Here's how the part is built. I have some questions about the finished solid (model axes, mm). Face numbers are marked on the shaded views. A direction names the side the tool comes from. Give positions to 0.01 mm unless a question says otherwise; leave off trailing zeros. Loops run counter-clockwise (first coordinate to the right, second up) from the corner with the lowest first, then second, coordinate; pieces in that order, holes last.
Q1. For the marked faces 1 and 2, which set-ups out of +Z, -Z, +X, -X, +Y, -Y let a thin tool reach every point of the face, with its end or its side?
Q2. Suppose I cut it at A-A (x = -25). List the corners of the cut face in (y, z) for me.
Q3. Suppose I cut it at D-D (y = -60.5). List the corners of the cut face in (x, z) for me, and give its area (3 significant figures).
Q4. Thinking about a two-plate mould opening in Z: for the marked faces 3, 4 and 5, which applies, pulls with the +Z half, pulls with the -Z half, needs draft (parallel to the pull), parting line crosses it, or undercut?
Q5. Suppose I cut it at C-C (z = -34). List the corners of the cut face in (x, y) for me, and give its area (3 significant figures).
Q6. I'm going to push flat-ended pins straight in: P1, Ø9, axis at x = -25, z = 0, coming from the +Y side; P2, Ø11, axis at x = 44.5, z = -45.5, coming from the +Y side; P3, Ø8, axis at x = 68.5, z = -7, coming from the -Y side; P4, Ø9, axis at x = 0, y = 0, coming from the -Z side. Where does each tip first touch, or does it pass through?
Q7. I need wall thicknesses on probe 1 along Y at (x, z) = (0, -49); probe 2 along Z at (x, y) = (-17, -44); probe 3 along X at (y, z) = (19.5, -35). Which ranges of each line are inside material? Lowest first, please.
Q8. Suppose I cut it at B-B (y = 35.5). List the corners of the cut face in (x, z) for me.
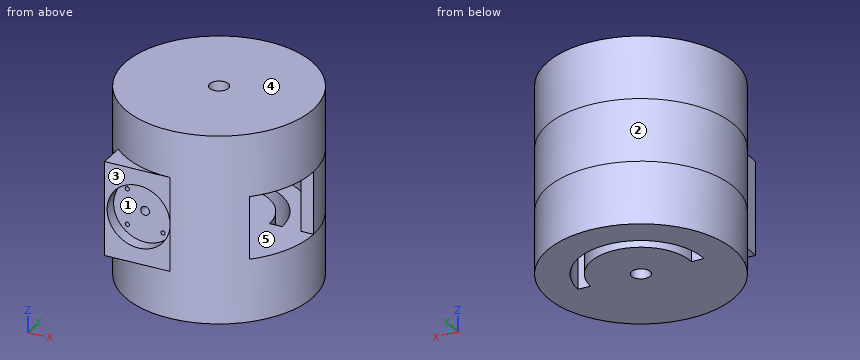
Autodesk Inventor part; units mm, degrees
ref_plane "Work Plane4" through (0, 0, 0) normal (0, 0, -1) x (-1, 0, 0)
ref_plane "YZ Plane" through (0, 0, 0) normal (1, 0, 0) x (0, 1, 0)
ref_plane "XZ Plane" through (0, 0, 0) normal (0, 1, 0) x (-1, 0, 0)
sketch "Sketch1" plane through (0, 0, 0) normal (0, 0, 1) x (1, 0, 0)
  circle A0 centre (0, 0) radius 75
  dimension "d0" = 150
extrude "Extrusion1" add sketch "Sketch1" along normal mid plane 150
sketch "Sketch32" plane through (0, 0, 0) normal (0, 0, 1) x (1, 0, 0)
  line L0 (0, 0) -> (-52, 0)
  line L1 (-52, 0) -> (-52, -75)
  line L2 (-52, -75) -> (0, -75)
  line L3 (0, -75) -> (0, 0)
  dimension "d94" = 52
  dimension "d95" = 75
extrude "Extrusion23" add sketch "Sketch32" along normal mid plane 75
sketch "Sketch39" plane through (0, 0, -75) normal (0, 0, -1) x (-1, 0, 0)
  circle A0 centre (0, 0) radius 7.5
  dimension "d141" = 15
extrude "Extrusion30" cut sketch "Sketch39" against normal through all
ref_plane "Work Plane4" through (0, 0, 0) normal (0, 0, -1) x (-1, 0, 0)
sketch "Sketch40" plane through (0, 0, 0) normal (0, 0, -1) x (-1, 0, 0)
  circle A0 centre (0, 0) radius 75
  dimension "d144" = 150
extrude "Extrusion31" cut sketch "Sketch40" along normal mid plane 50
sketch "Sketch41" plane through (0, 0, 0) normal (0, 0, -1) x (-1, 0, 0)
  line L0 (52, -75) -> (52, -54.0463)
  line L1 (52, -54.0463) -> (-52, -54.0463)
  circle A0 centre (0, 0) radius 75
  arc A1 (-52, -54.0463) -> (0, -75) centre (0, 0) ccw
extrude "Extrusion32" add sketch "Sketch41" along normal mid plane 50 contours A0 L1 picked at (-14.3807, -56.4807)
sketch "Sketch34" plane through (-52, -75, 37.5) normal (0, -1, 0) x (1, 0, 0)
  circle A0 centre (27, -37.5) radius 25
  line L0 (52, -75) -> (0, -75)
  line L1 (-23, -112.5) -> (127, -112.5)
  point P0 (52, -37.5)
  dimension "d104" = 50
  dimension "d105" = 25
  dimension "d106" = 37.5
extrude "Extrusion25" cut sketch "Sketch34" against normal blind 10
sketch "Sketch42" plane through (0, 0, 0) normal (0, 0, -1) x (-1, 0, 0)
  arc A0 (47, -44.8999) -> (1.9436, 64.9709) centre (0, 0) ccw
  line L0 (47, -44.8999) -> (47, -54.0463)
  line L1 (47, -54.0463) -> (52, -54.0463)
  arc A1 (52, -54.0463) -> (-75, 0) centre (0, 0) ccw
  arc A2 (47, -44.8999) -> (-65, 0) centre (0, 0) ccw
  line L2 (-65, 0) -> (-75, 0)
  line L3 (0, 0) -> (-92.1338, 0) construction
  dimension "d164" = 5
extrude "Extrusion33" add sketch "Sketch42" along normal mid plane 50
sketch "Sketch43" plane through (52, -54.0463, 25) normal (0, 1, 0) x (1, 0, 0)
  circle A0 centre (-77, 25) radius 25 construction
  line L0 (-62.8579, 10.8579) -> (-91.1421, 10.8579) construction
  line L1 (-91.1421, 10.8579) -> (-91.1421, 39.1421) construction
  line L2 (-91.1421, 39.1421) -> (-62.8579, 39.1421) construction
  line L3 (-62.8579, 39.1421) -> (-62.8579, 10.8579) construction
  line L4 (-62.8579, 10.8579) -> (-91.1421, 39.1421) construction
  line L5 (-91.1421, 10.8579) -> (-62.8579, 39.1421) construction
  circle A1 centre (-91.1421, 39.1421) radius 1.65
  circle A2 centre (-91.1421, 10.8579) radius 1.65
  circle A3 centre (-62.8579, 10.8579) radius 1.65
  circle A4 centre (-62.8579, 39.1421) radius 1.65
  circle A5 centre (-77, 25) radius 3.5
  line L6 (-52, 62.5) -> (-104, 62.5)
  line L7 (-52, 25) -> (-52, 62.5)
  point P0 (-75, 50)
  dimension "d154" = 50
  dimension "d155" = 28.2843
  dimension "d156" = 28.2843
  dimension "d157" = 3.3
  dimension "d158" = 3.3
  dimension "d159" = 3.3
  dimension "d160" = 3.3
  dimension "d163" = 7
  dimension "d165" = 37.5
  dimension "d166" = 25
extrude "Extrusion34" cut sketch "Sketch43" against normal through all
sketch "Sketch44" plane through (0, 0, -75) normal (0, 0, -1) x (-1, 0, 0)
  arc A0 (75, 0) -> (0, -75) centre (0, 0) ccw construction
  circle A1 centre (0, 0) radius 75
  line L0 (0, 0) -> (107.3838, 0) construction
  arc A2 (50, 0) -> (-50, 0) centre (0, 0) ccw
  arc A3 (40, 0) -> (-40, 0) centre (0, 0) ccw
  line L1 (40, 0) -> (50, 0)
  line L2 (0, -55) -> (0, -55.9017)
  line L3 (-52, -54.0463) -> (47, -54.0463)
  line L4 (0, -75) -> (52, -75)
  line L5 (-50, 0) -> (-40, 0)
  dimension "d167" = 25
  dimension "d168" = 10
extrude "Extrusion35" cut sketch "Sketch44" against normal blind 50 contours L1 A3 L5 A2
properties material "ABS Plastic"
Solutions:
1. face 1: -Y
1. face 2: +Z, -Z
2. outline: (-75, -37.5) - (-70.71, -37.5) - (-70.71, -75) - (31.22, -75) - (31.22, -25) - (-54.05, -25) - (-54.05, -3.5) - (-65, -3.5) - (-65, -25) - (-75, -25) - close; (-75, 25) - (-65, 25) - (-65, 3.5) - (-54.05, 3.5) - (-54.05, 25) - (60, 25) - (60, -25) - (43.3, -25) - (43.3, -75) - (70.71, -75) - (70.71, 25) - (70.71, 75) - (-70.71, 75) - (-70.71, 37.5) - (-75, 37.5) - close
3. outline: (-52, -37.5) - (-44.33, -37.5) - (-44.33, -75) - (44.33, -75) - (44.33, 75) - (-44.33, 75) - (-44.33, 37.5) - (-52, 37.5) - close; hole circle Ø3.3 at (-39.14, -14.14); hole circle Ø3.3 at (-39.14, 14.14); hole circle Ø7 at (-25, 0); hole circle Ø3.3 at (-10.86, -14.14); hole circle Ø3.3 at (-10.86, 14.14)
3. area: 13,800 mm2
4. face 3: needs draft
4. face 4: pulls with the +Z half
4. face 5: undercut
5. outline: (-52, -75) - (0, -75) arc R75 ccw (long way) to (-52, -54.05) - close; hole (-50, 0) - (-40, 0) arc R40 cw to (40, 0) - (50, 0) arc R50 ccw to start; hole circle Ø15 at (0, 0)
5. area: 16,400 mm2
6. P1: stops at y = 72.14
6. P2: stops at y = 64.06
6. P3: stops at y = 0
6. P4: passes through
7. probe 1: y = -75 to -7.5, 7.5 to 40, 50 to 75
7. probe 2: z = -75 to -25, 25 to 75
7. probe 3: x = -72.42 to -46.04, -34.92 to 34.92, 46.04 to 72.42
8. outline: (-66.07, -75) - (-35.21, -75) - (-35.21, -25) - (-54.45, -25) - (-54.45, 25) - (54.45, 25) - (54.45, -25) - (35.21, -25) - (35.21, -75) - (66.07, -75) - (66.07, 75) - (-66.07, 75) - (-66.07, 25) - close; (-18.43, -75) - (18.43, -75) - (18.43, -25) - (-18.43, -25) - close
